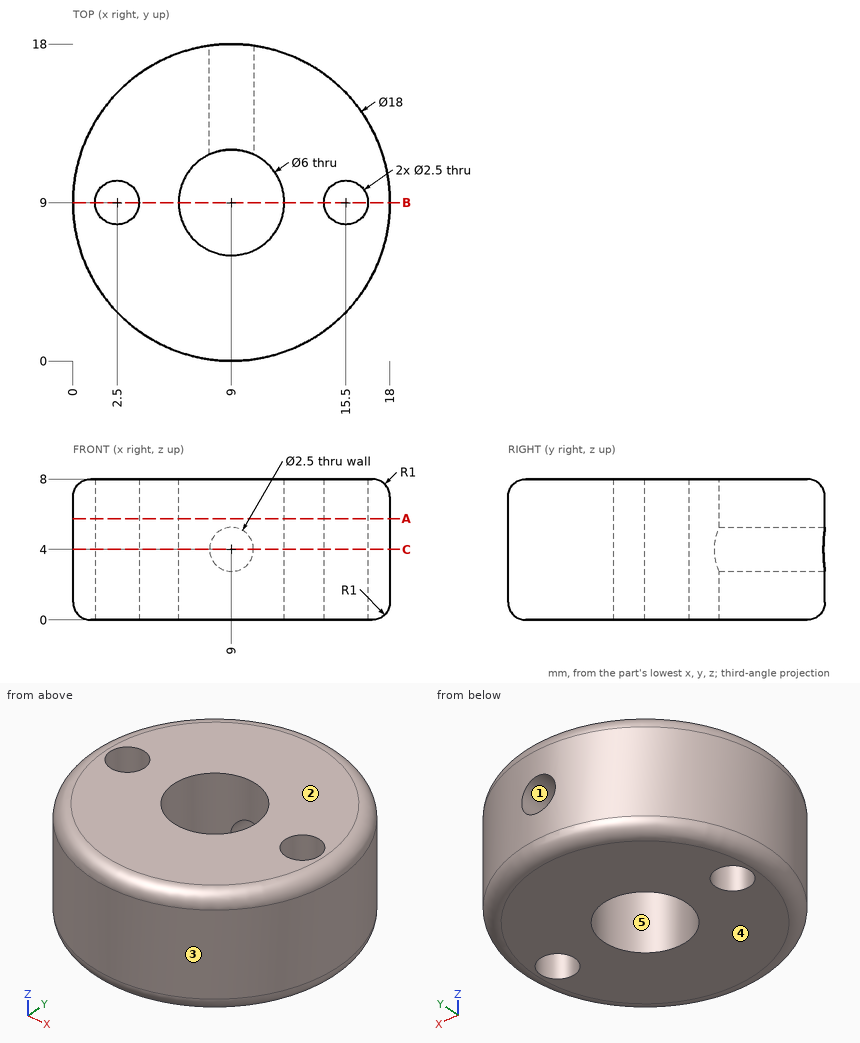
Here's the drawing with two shaded views (mm, measured from the low corner). I have some questions. A direction names the side the tool comes from. Give positions to 0.01 mm unless a question says otherwise; leave off trailing zeros. Write each loop counter-clockwise with the first axis right and the second up, starting at its lowest first coordinate (ties: lowest second). Pieces come first, ordered by that corner, then holes. Notation, with made-up numbers: (16, -3.5) -> (66, -3.5) arc R32 cw to (66, 26.5) -> close; hole circle Ø7 at (59.5, -23.5). An arc over 180 degrees is marked (long way). One line per item, written item: value.
Q1. For P1, Ø1, axis at y = 6, z = 5, coming from the +X side; P2, Ø1.5, axis at y = 15, z = 1, coming from the +X side; P3, Ø4, axis at y = 6.5, z = 4, coming from the +X side, each with a flat end and sliding along its axis, tell me the tip position at first contact or that it passes through.
Results found:
P1: stops at x = 17.65
P2: stops at x = 16.31
P3: stops at x = 17.99
Q2. Imagine slicing it at C-C on z = 4. Please give me the cut outline in (x, y), and give its area (3 significant figures).
Results found:
outline: (7.75, 11.73) -> (7.75, 17.91) arc R9 ccw (long way) to (10.25, 17.91) -> (10.25, 11.73) arc R3 cw (long way) to start; hole circle Ø2.5 at (2.5, 9); hole circle Ø2.5 at (15.5, 9)
area: 201 mm^2
Q3. Please list where these lines run through material, in increasing order: line 1 (Z direction, x = 9, y = 14.5); line 2 (X direction, y = 9.75, z = 3.5); line 3 (Y direction, x = 15.5, z = 3). Write a range as [from, to].
Results found:
line 1: z = [0, 2.75], [5.25, 8]
line 2: x = [0.03, 1.5], [3.5, 6.1], [11.9, 14.5], [16.5, 17.97]
line 3: y = [2.78, 7.75], [10.25, 15.22]
Q4. Which directions (+Z, -Z, +X, -X, +Y, -Y) give clear straight access to the entire face, cutting with the end or side of a thin tool? Please do the marked faces 1 and 2.
Results found:
face 1: +Y
face 2: +Z, +X, -X, +Y, -Y
Q5. We'd pull the mould along X, two halves only. Please class the marked faces 3, 4 and 5: +X half, -X half, draft (parallel to the pull), parting line (faces both ways), or undercut.
Results found:
face 3: parting line
face 4: draft
face 5: undercut
Q6. Imagine slicing it at A-A on z = 5.75. Please give me the cut outline in (x, y).
Results found:
outline: circle Ø18 at (9, 9); hole circle Ø2.5 at (2.5, 9); hole circle Ø6 at (9, 9); hole circle Ø2.5 at (15.5, 9)
Q7. Imagine slicing it at B-B on y = 9. Give the number of separate pieces and of enclosed holes in the cut face, and give its area (3 significant figures).
Results found:
separate pieces: 4
enclosed holes: 0
area: 55.1 mm^2
